Model file for the job. Use its own axes, mm. A direction names the side the tool comes from. Give positions to 0.01 mm unless a question says otherwise; leave off trailing zeros. Loops run counter-clockwise (first coordinate to the right, second up) from the corner with the lowest first, then second, coordinate; pieces in that order, holes last. Notation, with made-up numbers: M 10.5,60 L 45.5,60 A19 cw 45.5,85 Z; hole C 76.5,49.25 d10. An arc over 180 degrees is marked long. Answer in a Markdown table with one row per item.
Autodesk Inventor part; units mm, degrees
ref_plane "P21_XY" through (0, 20, 0) normal (0, 0, -1) x (1, 0, 0)
ref_plane "P21_YZ" through (0, 20, 0) normal (1, 0, 0) x (0, -1, 0)
ref_plane "P21_ZX" through (0, 20, 0) normal (0, -1, 0) x (0, 0, -1)
sketch "Sketch_8" plane through (0, 0, 0) normal (0, 0, 1) x (1, 0, 0)
  line L0 (-37, 26) -> (-37, -26)
  line L1 (-37, -26) -> (-31, -32)
  line L2 (-31, -32) -> (16, -32)
  line L3 (16, -32) -> (16, 32)
  line L4 (16, 32) -> (-31, 32)
  line L5 (-31, 32) -> (-37, 26)
  circle A0 centre (0, -20) radius 5.5
  circle A1 centre (0, 20) radius 5.5
  circle A2 centre (-25, -20) radius 5.5
  circle A3 centre (-25, 20) radius 5.5
extrude "Extrusion1" add sketch "Sketch_8" against normal blind 3
sketch "Sketch_1" plane through (0, 0, 0) normal (0, 1, 0) x (1, 0, 0)
  arc A0 (20, -4) -> (16, 0) centre (16, -4) ccw
  line L0 (20, -4) -> (23, -4)
  arc A1 (23, -4) -> (16, 3) centre (16, -4) ccw
  line L1 (16, 3) -> (16, 0)
extrude "Extrusion2" add sketch "Sketch_1" along normal mid plane 64
sketch "Sketch_2" plane through (23, 0, 0) normal (1, 0, 0) x (0, 0, -1)
  line L0 (-22, -30) -> (-20, -32)
  line L1 (-20, -32) -> (-4, -32)
  line L2 (-4, -32) -> (-4, 32)
  line L3 (-4, 32) -> (-20, 32)
  line L4 (-20, 32) -> (-22, 30)
  line L5 (-22, 30) -> (-22, -30)
  circle A0 centre (-15, -25) radius 4.25
  circle A1 centre (-15, -12.5) radius 4.25
  circle A2 centre (-15, 0) radius 4.25
  circle A3 centre (-15, 12.5) radius 4.25
  circle A4 centre (-15, 25) radius 4.25
extrude "Extrusion3" add sketch "Sketch_2" against normal blind 3
ref_plane "P21_XY" through (0, 20, 0) normal (0, 0, -1) x (1, 0, 0)
ref_plane "P21_YZ" through (0, 20, 0) normal (1, 0, 0) x (0, -1, 0)
ref_plane "P21_ZX" through (0, 20, 0) normal (0, -1, 0) x (0, 0, -1)
ref_plane "P22_XY" through (0, -20, 0) normal (0, 0, -1) x (1, 0, 0)
ref_plane "P22_YZ" through (0, -20, 0) normal (1, 0, 0) x (0, -1, 0)
ref_plane "P22_ZX" through (0, -20, 0) normal (0, -1, 0) x (0, 0, -1)
properties part number "8617.540_P2"
(1) Saw through at C-C, the plane y = 0. Give the cut face in (x, z).
Established:
| item | result |
|---|---|
| outline | M -37,-3 L 16,-3 A7 ccw 23,4 L 23,10.75 L 20,10.75 L 20,4 A4 cw 16,0 L -37,0 Z; M 20,19.25 L 23,19.25 L 23,22 L 20,22 Z |
(2) Mould opens along Z. For faces 3 (the cylindrical face through (21.521, 28.584, 12.715)), 4 (the flat face through (-11, 0, -3)), 5 (the cylindrical face through (-22.043, 24.638, -1.479)) say: pulls with the +Z half, pulls with the -Z half, needs draft (parallel to the pull), parting line crosses it, or undercut.
Established:
| item | result |
|---|---|
| face 3 | undercut |
| face 4 | pulls with the -Z half |
| face 5 | needs draft |
(3) Which spindle directions (+Z, -Z, +X, -X, +Y, -Y) get a long thin tool onto all of the face, cutting with end or side? Do faces 1 (the flat face through (20, 0, 9)), 2 (the flat face through (22, -31, 21)). Say none if no direction does.
Established:
| item | result |
|---|---|
| face 1 | +Z, -X, +Y, -Y |
| face 2 | +Z, +X, -X, -Y |
(4) Saw through at A-A, the plane x = -25. Give the cut face in (y, z), and give its area (3 significant figures).
Established:
| item | result |
|---|---|
| outline | M -32,-3 L -25.5,-3 L -25.5,0 L -32,0 Z; M -14.5,-3 L 14.5,-3 L 14.5,0 L -14.5,0 Z; M 25.5,-3 L 32,-3 L 32,0 L 25.5,0 Z |
| area | 126 mm2 |
(5) Saw through at D-D, the plane z = 15. Give the cut face in (x, y).
Established:
| item | result |
|---|---|
| outline | M 20,-32 L 23,-32 L 23,-29.25 L 20,-29.25 Z; M 20,-20.75 L 23,-20.75 L 23,-16.75 L 20,-16.75 Z; M 20,-8.25 L 23,-8.25 L 23,-4.25 L 20,-4.25 Z; M 20,4.25 L 23,4.25 L 23,8.25 L 20,8.25 Z; M 20,16.75 L 23,16.75 L 23,20.75 L 20,20.75 Z; M 20,29.25 L 23,29.25 L 23,32 L 20,32 Z |
(6) Saw through at B-B, the plane y = 20. Give the cut face in (x, z).
Established:
| item | result |
|---|---|
| outline | M -37,-3 L -30.5,-3 L -30.5,0 L -37,0 Z; M -19.5,-3 L -5.5,-3 L -5.5,0 L -19.5,0 Z; M 5.5,-3 L 16,-3 A7 ccw 23,4 L 23,22 L 20,22 L 20,4 A4 cw 16,0 L 5.5,0 Z |
(7) Wall check: L1, parallel to Y at x = 20.95, z = 15; L2, parallel to X at y = 24.5, z = -0.5; L3, parallel to Z at x = -6, y = 26.5. Give the ranges that are in metal, low to high.
Established:
| item | result |
|---|---|
| L1 | y = -32 to -29.25, -20.75 to -16.75, -8.25 to -4.25, 4.25 to 8.25, 16.75 to 20.75, 29.25 to 32 |
| L2 | x = -37 to -28.16, -21.84 to -3.16, 3.16 to 21.36 |
| L3 | z = -3 to 0 |
(8) Flat gauge pins, fed straight in: P1, Ø9, axis at x = 0, y = 20, coming from the -Z side; P2, Ø10, axis at y = -12.5, z = 15, coming from the +X side; P3, Ø9, axis at y = -12.5, z = 17, coming from the -X side; P4, Ø8, axis at x = 14, y = 11, coming from the +Z side. Where does each tip first touch, or does it go through?
Established:
| item | result |
|---|---|
| P1 | passes through |
| P2 | stops at x = 23 |
| P3 | stops at x = 20 |
| P4 | stops at z = 0.54 |
